from build123d import *

# Parameters (mm, degrees)
SKETCH_1_W          = 30
SKETCH_1_H          = 30
EXTRUDE_1_DEPTH     = 10
CUT_EXTRUDE_1_REACH = 45.589
SKETCH_2_R          = 5
FILLET_1_R          = 7
SKETCH_3_R          = 3
CUT_EXTRUDE_2_DEPTH = 12


with BuildPart() as part:
    # 草图1 → 凸台-拉伸1 (new body)
    with BuildSketch(Plane.XY):
        with Locations((15, 15)):
            Rectangle(SKETCH_1_W, SKETCH_1_H)
    extrude(amount=EXTRUDE_1_DEPTH)

    # 草图2 → 切除-拉伸1 (cut, up to next)
    with BuildSketch(Plane(origin=(0, 0, 0), x_dir=(-1, 0, 0), z_dir=(0, 0, -1)), mode=Mode.PRIVATE) as cut_extrude_1_sk1:
        with Locations((-21, 15)):
            Circle(SKETCH_2_R)
    cut_extrude_1_tool1 = extrude(cut_extrude_1_sk1.sketch, amount=-CUT_EXTRUDE_1_REACH, mode=Mode.PRIVATE) & part.part
    add(cut_extrude_1_tool1.solids().sort_by_distance((21, 15, 0))[0], mode=Mode.SUBTRACT)

    # 圆角1
    fillet_1_edges = [part.edges().sort_by_distance(p)[0] for p in [
        (0, 30, 5),
        (30, 30, 5),
        (30, 0, 5),
        (0, 0, 5),
    ]]
    fillet(fillet_1_edges, radius=FILLET_1_R)

    # 草图3 → 切除-拉伸2 (cut)
    with BuildSketch(Plane.ZY):
        with Locations((5, 15)):
            Circle(SKETCH_3_R)
    extrude(amount=-CUT_EXTRUDE_2_DEPTH, mode=Mode.SUBTRACT)


solid = part.part
Work out the finished part from the listing and answer in its coordinate system (mm). A direction names the side the tool comes from. Give positions to 0.01 mm unless a question says otherwise; leave off trailing zeros. Loops run counter-clockwise (first coordinate to the right, second up) from the corner with the lowest first, then second, coordinate; pieces in that order, holes last. Notation, with made-up numbers: (-33, 0.25) -> (-5, 0.25) arc R25 cw to (-5, 16.25) -> close; hole circle Ø6 at (36.25, 66.5). An arc over 180 degrees is marked (long way). Use a Markdown table: item, result. Add a question column.
1) The part is cut by section B-B, the plane y = 15. Determine the outline of the cut face in (x, z).
2) The part is cut by section C-C, the plane z = 5. Determine the outline of the cut face in (x, y), plus the area to 3 significant figures.
3) Which of the six approach directions +Z, -Z, +X, -X, +Y, -Y give full straight-line access (tool end or side, diameter ignored) to faces 1 (the cylindrical face through (5.92, 12.07, 4.35)), 2 (the cylindrical face through (27.9, 2, 5.1))?
4) Consider line 1 along Y through (x, z) = (9.75, 5); line 2 along Y through (x, z) = (21, 3.75); line 3 along Z through (x, y) = (4.25, 14). Determine where each line is inside the solid, lowest interval first.
5) This flat-tipped pin is pushed along its axis until it touches: P1, Ø4, axis at x = 26.5, z = 5, coming from the +Y side. Where does it stop, or does it pass through?
6) For a pull along X with two mould halves and no side action, classify faces 3 (the cylindrical face through (27.9, 28, 5.1)), 4 (the flat face through (15, 30, 5)), 5 (the cylindrical face through (2, 2.1, 5.1)), 6 (the cylindrical face through (22.08, 10.12, 4.93)) as +X half, -X half, draft (parallel to the pull), parting line (faces both ways), or undercut.
7) The part is cut by section A-A, the plane x = 21. Determine the outline of the cut face in (y, z), plus the area to 3 significant figures.
8) The part is cut by section D-D, the plane z = 1. Determine the outline of the cut face in (x, y).
Reported:
| question | item | result |
|---|---|---|
| 1 | outline | (0, 0) -> (16, 0) -> (16, 10) -> (0, 10) -> (0, 8) -> (12, 8) -> (12, 2) -> (0, 2) -> close; (26, 0) -> (30, 0) -> (30, 10) -> (26, 10) -> close |
| 2 | outline | (0, 7) arc R7 ccw to (7, 0) -> (23, 0) arc R7 ccw to (30, 7) -> (30, 23) arc R7 ccw to (23, 30) -> (7, 30) arc R7 ccw to (0, 23) -> (0, 18) -> (12, 18) -> (12, 12) -> (0, 12) -> close; hole circle Ø10 at (21, 15) |
| 2 | area | 707 mm^2 |
| 3 | face 1 | -X |
| 3 | face 2 | +Z, -Z, +X, -Y |
| 4 | line 1 | y = 0 to 12, 18 to 30 |
| 4 | line 2 | y = 0 to 10, 20 to 30 |
| 4 | line 3 | z = 0 to 2.17, 7.83 to 10 |
| 5 | P1 | stops at y = 29.84 |
| 6 | face 3 | +X half |
| 6 | face 4 | draft |
| 6 | face 5 | -X half |
| 6 | face 6 | undercut |
| 7 | outline | (0, 0) -> (10, 0) -> (10, 10) -> (0, 10) -> close; (20, 0) -> (30, 0) -> (30, 10) -> (20, 10) -> close |
| 7 | area | 200 mm^2 |
| 8 | outline | (0, 7) arc R7 ccw to (7, 0) -> (23, 0) arc R7 ccw to (30, 7) -> (30, 23) arc R7 ccw to (23, 30) -> (7, 30) arc R7 ccw to (0, 23) -> close; hole circle Ø10 at (21, 15) |
